from build123d import *

# Parameters (mm, degrees)
ESQUISSE1_W                                     = 10
ESQUISSE1_H                                     = 10
BOSS_EXTRU_1_DEPTH                              = 79
ESQUISSE2_R                                     = 3.75
ESQUISSE2_R_2                                   = 1.75
BOSS_EXTRU_2_DEPTH                              = 30
R_P_TITION_LIN_AIRE1_COUNT                      = 3
R_P_TITION_LIN_AIRE1_PITCH                      = 64
CHAMBRAGE_POUR_VIS_T_TE_CYLINDRIQUE_D           = 3.4
CHAMBRAGE_POUR_VIS_T_TE_CYLINDRIQUE_CBORE_D     = 6.5
CHAMBRAGE_POUR_VIS_T_TE_CYLINDRIQUE_CBORE_DEPTH = 3
CHANFREIN1_SIZE                                 = 2.5


with BuildPart() as part:
    # Esquisse1 → Boss.-Extru.1 (new, symmetric)
    with BuildSketch(Plane.XY):
        Rectangle(ESQUISSE1_W, ESQUISSE1_H)
    extrude(amount=BOSS_EXTRU_1_DEPTH, both=True)

    # Esquisse2 → Boss.-Extru.2 (add)
    # profile 1 of 3: a face of its own
    with BuildSketch(Plane(origin=(0, 0, -79), x_dir=(-1, 0, 0), z_dir=(0, 0, -1))):
        with BuildLine():
            Line((-5, 5), (-1.25, 5))
            ThreePointArc((-1.25, 5), (-3.901650429, 6.098349571), (-5, 8.75))
            Line((-5, 8.75), (-5, 5))
        make_face()
    # profile 2 of 3: a face of its own
    with BuildSketch(Plane(origin=(0, 0, -79), x_dir=(-1, 0, 0), z_dir=(0, 0, -1))):
        with Locations((-1.25, 8.75)):
            Circle(ESQUISSE2_R)
        with Locations((-1.25, 8.75)):
            Circle(ESQUISSE2_R_2, mode=Mode.SUBTRACT)
    # profile 3 of 3: a face of its own
    with BuildSketch(Plane(origin=(0, 0, -79), x_dir=(-1, 0, 0), z_dir=(0, 0, -1))):
        with BuildLine():
            ThreePointArc((2.5, 8.75), (1.401650429, 6.098349571), (-1.25, 5))
            Line((-1.25, 5), (2.5, 5))
            Line((2.5, 5), (2.5, 8.75))
        make_face()
    boss_extru_2 = extrude(amount=-BOSS_EXTRU_2_DEPTH)

    # Répétition linéaire1: Boss.-Extru.2 ×3
    with Locations(*[(0, 0, i * R_P_TITION_LIN_AIRE1_PITCH) for i in range(1, R_P_TITION_LIN_AIRE1_COUNT)]):
        add(boss_extru_2)

    # Chambrage pour vis à tête cylindrique à 6 pans creux (ou vis CHC) M31 (through all)
    with Locations(Plane(origin=(5, 0, 0), x_dir=(0, 0, -1), z_dir=(1, 0, 0))):
        with Locations((-75, 0), (75, 0)):
            CounterBoreHole(CHAMBRAGE_POUR_VIS_T_TE_CYLINDRIQUE_D / 2, CHAMBRAGE_POUR_VIS_T_TE_CYLINDRIQUE_CBORE_D / 2, CHAMBRAGE_POUR_VIS_T_TE_CYLINDRIQUE_CBORE_DEPTH)

    # Chanfrein1
    chanfrein1_edges = [part.edges().sort_by_distance(p)[0] for p in [
        (-2.5, 5, 64),
        (-2.5, 5, 0),
        (-2.5, 5, -64),
    ]]
    chamfer(chanfrein1_edges, length=CHANFREIN1_SIZE - 0.0001)  # a hair under: the kernel refuses the full size


solid = part.part
For this review, take the finished solid that the model builds, in its own axes (mm). A direction names the side the tool comes from. Give positions to 0.01 mm unless a question says otherwise; leave off trailing zeros. Order: outer loops, then holes, each group sorted by start corner. A loop starts at its lowest first (then second) coordinate and runs counter-clockwise, first axis right, second up. Notation, with made-up numbers: (40.5, 47) -> (66.5, 47) arc R15 ccw to (66.5, 73) -> close; hole circle Ø10 at (44, 29.5). An arc over 180 degrees is marked (long way). Write item = value, one per line.
1) To check wall thickness, follow L1, parallel to Z at x = 4.25, y = 6; L2, parallel to Z at x = 4.5, y = -1.5; L3, parallel to Y at x = 1.25, z = 61.5. State the ranges of each line that lie inside material, in increasing order. Write a range as from..to.
Findings:
L1 = -79..-49, -15..15, 49..79
L2 = -79..-77.88, -72.12..72.12, 77.88..79
L3 = -5..7, 10.5..12.5
2) For faces 1 (the face through (2, -1.4, -76.4)), 2 (the face through (0, 7, 49)), 3 (the face through (1.478, 10.485, -64.21)), list the 3-axis set-ups (+Z, -Z, +X, -X, +Y, -Y) from which the entire face can be reached by the end or side of a thin tool; tool diameter is ignored.
Findings:
face_1 = +X
face_2 = +X, -X, +Y
face_3 = +Z, -Z
3) We need section B-B, the plane y = 0. Give the boundary of the cut face in (x, z), and give its area (3 significant figures).
Findings:
outline = (-5, -79) -> (5, -79) -> (5, -78.25) -> (2, -78.25) -> (2, -76.7) -> (-5, -76.7) -> close; (-5, -73.3) -> (2, -73.3) -> (2, -71.75) -> (5, -71.75) -> (5, 71.75) -> (2, 71.75) -> (2, 73.3) -> (-5, 73.3) -> close; (-5, 76.7) -> (2, 76.7) -> (2, 78.25) -> (5, 78.25) -> (5, 79) -> (-5, 79) -> close
area = 1,490 mm^2
4) Draft analysis for pull direction Y (two halves, no side actions). For faces 4 (the face through (-1.55, 0.07, 73.3)), 5 (the face through (0, 5, 19)), 6 (the face through (0, 7, 15)), 7 (the face through (0, -5, 1)), state which applies: pulls with the +Y half, pulls with the -Y half, needs draft (parallel to the pull), parting line crosses it, or undercut.
Findings:
face_4 = undercut
face_5 = pulls with the +Y half
face_6 = needs draft
face_7 = pulls with the -Y half
5) We need section A-A, the plane z = -75. Count the separate pieces of the cut face and the enclosed holes in it, and give its area (3 significant figures).
Findings:
separate_pieces = 2
enclosed_holes = 1
area = 100 mm^2
6) We need section D-D, the plane z = -34. Give the boundary of the cut face in (x, y), and give its area (3 significant figures).
Findings:
outline = (-5, -5) -> (5, -5) -> (5, 5) -> (-5, 5) -> close
area = 100 mm^2
